The listing builds one solid part. Answer for the finished solid, in the listing's coordinates (mm). A direction names the side the tool comes from. Coordinates: 2 decimals unless noted, no trailing zeros. Loops run counter-clockwise (first coordinate to the right, second up) from the corner with the lowest first, then second, coordinate; pieces in that order, holes last. Notation, with made-up numbers: M 10,1 L 31,1 A10 ccw 31,13 Z; hole C 20,45 d11. An arc over 180 degrees is marked long. Answer as a JSON object with one key per item and string values. Group by question number.
1. A cutting plane is placed at B-B on z = 5.25. Give the vertices of the cut face in (x, y), and give its area (3 significant figures).
2. A cutting plane is placed at A-A on y = 0. Give the vertices of the cut face in (x, z) (3 decimals).
3. A cutting plane is placed at D-D on y = 8.75. Give the vertices of the cut face in (x, z), and give its area (3 significant figures).
4. For faces 1 (the face through (-5, -2, 6.5)), 2 (the face through (1.08, -4.88, 3.2)), determine the directions among +Z, -Z, +X, -X, +Y, -Y from which every point of the face is accessible in a straight line to the end or side of a thin tool.
5. A cutting plane is placed at C-C on y = -3. Give the vertices of the cut face in (x, z), and give its area (3 significant figures).
6. Determine the mould class of faces 3 (the face through (67.5, -0.16, 4.93)), 4 (the face through (27, 0, 0)), 5 (the face through (9.9, 3.1, 8.3)) for opening direction X: released by +X, released by -X, zero draft, split by the parting line, or undercut.
7. Given pin 1 (1 mm diameter, centred on y = 4, z = 4, fed in from +X); pin 2 (6 mm diameter, centred on x = -3, y = 4.5, fed in from +Z); pin 3 (1.5 mm diameter, centred on y = 3, z = 1, fed in from +X); pin 4 (9 mm diameter, centred on x = 0, y = 0, fed in from +Z), each flat-ended and moving along its own axis, determine where each tip first touches the part or whether it passes through.
8. Straight lines are drawn through the part: L1, parallel to Y at x = 0, z = 4.5; L2, parallel to Y at x = 0, z = 8.2 (3 decimals); L3, parallel to X at y = -3, z = 0.5. For each, find the intervals that lie inside material, in ascending order.
from build123d import *

# Parameters (mm, degrees)
EXTRUDE_1_DEPTH     = 10
SKETCH_2_R          = 10.375
CUT_EXTRUDE_1_DEPTH = 3.5
SKETCH_3_R          = 5
CUT_EXTRUDE_2_DEPTH = 70.283836499


with BuildPart() as part:
    # 草图1 → 凸台-拉伸1 (new body)
    with BuildSketch(Plane.XY):
        with BuildLine():
            Line((0.9, -11.966202405), (60.5625, -7.478876503))
            ThreePointArc((60.5625, -7.478876503), (67.5, 0), (60.5625, 7.478876503))
            Line((60.5625, 7.478876503), (0.9, 11.966202405))
            ThreePointArc((0.9, 11.966202405), (-12, 0), (0.9, -11.966202405))
        make_face()
    extrude(amount=EXTRUDE_1_DEPTH)

    # 草图2 → 切除-拉伸1 (cut)
    with BuildSketch(Plane.XY.offset(10)):
        Circle(SKETCH_2_R)
    extrude(amount=-CUT_EXTRUDE_1_DEPTH, mode=Mode.SUBTRACT)

    # 草图3 → 切除-拉伸2 (cut, through all)
    with BuildSketch(Plane(origin=(0, 0, 0), x_dir=(-1, 0, 0), z_dir=(0, 0, -1))):
        Circle(SKETCH_3_R)
    extrude(amount=-CUT_EXTRUDE_2_DEPTH, mode=Mode.SUBTRACT)


solid = part.part
From the geometry:
{
 "1": {"outline": "M 0.9,-11.97 L 60.56,-7.48 A7.5 ccw 60.56,7.48 L 0.9,11.97 A12 ccw long Z; hole C 0,0 d10", "area": "1,410 mm²"},
 "2": {"outline": "M -12,0 L -5,0 L -5,6.5 L -10.375,6.5 L -10.375,10 L -12,10 Z; M 5,0 L 67.5,0 L 67.5,10 L 10.375,10 L 10.375,6.5 L 5,6.5 Z"},
 "3": {"outline": "M -8.21,0 L 43.66,0 L 43.66,10 L 5.57,10 L 5.57,6.5 L -5.57,6.5 L -5.57,10 L -8.21,10 Z", "area": "480 mm²"},
 "4": {"face 1": "+Z", "face 2": "+Z, -Z"},
 "5": {"outline": "M -11.62,0 L -4,0 L -4,6.5 L -9.93,6.5 L -9.93,10 L -11.62,10 Z; M 4,0 L 66.87,0 L 66.87,10 L 9.93,10 L 9.93,6.5 L 4,6.5 Z", "area": "663 mm²"},
 "6": {"face 3": "released by +X", "face 4": "zero draft", "face 5": "undercut"},
 "7": {"pin 1": "stops at x = 66.63", "pin 2": "stops at z = 6.5", "pin 3": "stops at x = 67.15", "pin 4": "passes through"},
 "8": {"L1": "y = -12 to -5, 5 to 12", "L2": "y = -12 to -10.375, 10.375 to 12", "L3": "x = -11.62 to -4, 4 to 66.87"}
}
